Source: three-view drawing plus pictorial views. Frame: mm from the lowest corner of the part. A direction names the side the tool comes from. Coordinates: 2 decimals unless noted, no trailing zeros. Write each loop counter-clockwise with the first axis right and the second up, starting at its lowest first coordinate (ties: lowest second). Pieces come first, ordered by that corner, then holes. Notation, with made-up numbers: (65, -6) - (80, -6) arc R19 ccw to (80, 29) - close; hole circle Ø11 at (33, 74.5). An arc over 180 degrees is marked (long way). One line per item, written item: value.
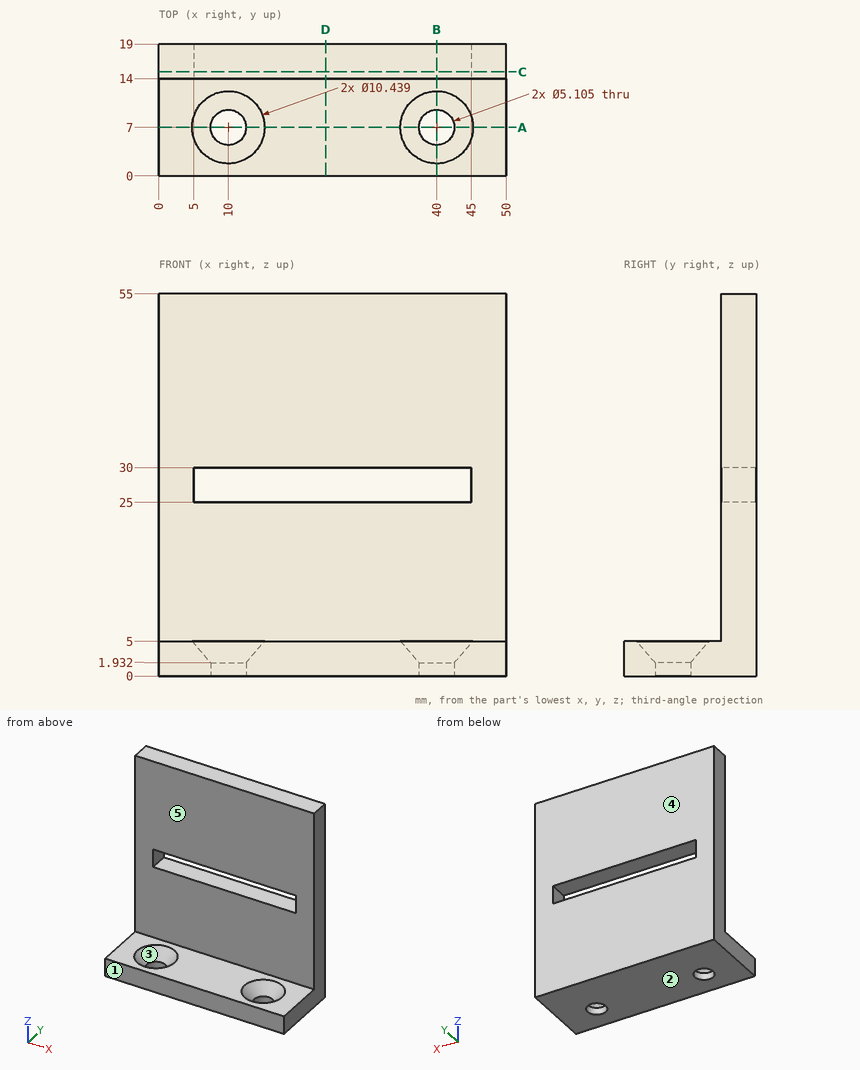
1) Reachability of the marked faces 4 and 5 from +Z, -Z, +X, -X, +Y, -Y: full face, straight path, thin tool, end or side. Return the list, or none.
Values found:
face 4: +Z, -Z, +X, -X, +Y
face 5: +Z, +X, -X, -Y
2) Section query C-C on y = 15. Output: boundary loops of the cut face in (x, z), then the cut area to 3 significant figures.
Values found:
outline: (0, 0) - (50, 0) - (50, 55) - (0, 55) - close; hole (5, 25) - (45, 25) - (45, 30) - (5, 30) - close
area: 2,550 mm2
3) Contact query for flat-ended pins moving along their axis: P1, Ø15, axis at x = 15.5, z = 30.5, coming from the -Y side; P2, Ø1, axis at y = 12, z = 18.5, coming from the -X side. Output: stop coordinate, or through.
Values found:
P1: y = 14
P2: through
4) Material intervals for line 1 (X direction, y = 7, z = 1.2); line 2 (Y direction, x = 10, z = 1.4); line 3 (Z direction, x = 6, y = 17.75), sorted ascending.
Values found:
line 1: 0 to 7.45, 12.55 to 37.45, 42.55 to 50
line 2: 0 to 4.45, 9.55 to 19
line 3: 0 to 25, 30 to 55
5) Draft query along Y for the marked faces 1, 2 and 3. Return one class per face: released by +Y, released by -Y, zero draft, split by the parting line, or undercut.
Values found:
face 1: released by -Y
face 2: zero draft
face 3: undercut
6) Section query D-D on x = 24. Output: boundary loops of the cut face in (y, z), then the cut area to 3 significant figures.
Values found:
outline: (0, 0) - (19, 0) - (19, 25) - (14, 25) - (14, 5) - (0, 5) - close; (14, 30) - (19, 30) - (19, 55) - (14, 55) - close
area: 320 mm2
7) Section query B-B on x = 40. Output: boundary loops of the cut face in (y, z).
Values found:
outline: (0, 0) - (4.45, 0) - (4.45, 1.93) - (1.78, 5) - (0, 5) - close; (9.55, 0) - (19, 0) - (19, 25) - (14, 25) - (14, 5) - (12.22, 5) - (9.55, 1.93) - close; (14, 30) - (19, 30) - (19, 55) - (14, 55) - close
8) Section query A-A on y = 7. Output: boundary loops of the cut face in (x, z).
Values found:
outline: (0, 0) - (7.45, 0) - (7.45, 1.93) - (4.78, 5) - (0, 5) - close; (12.55, 0) - (37.45, 0) - (37.45, 1.93) - (34.78, 5) - (15.22, 5) - (12.55, 1.93) - close; (42.55, 0) - (50, 0) - (50, 5) - (45.22, 5) - (42.55, 1.93) - close
